```python
from build123d import *

# Parameters (mm, degrees)
SKETCH1_R             = 66.4845
BOSS_EXTRUDE1_DEPTH   = 11.43
CUT_EXTRUDE1_START    = -33.02
SKETCH3_W             = 41.275
SKETCH3_H             = 24.257
CUT_EXTRUDE1_DEPTH    = 46.278900076
SKETCH4_R             = 30.1625
CUT_EXTRUDE2_DEPTH    = 95.715481208
F_6_CLEARANCE_HOLE1_D = 3.7973
CIRPATTERN1_COUNT     = 5
CUT_EXTRUDE3_DEPTH    = 95.715481208
SKETCH9_W             = 90.169443187
SKETCH9_H             = 19.134747519
CUT_EXTRUDE4_DEPTH    = 82.281975988
CUT_EXTRUDE5_DEPTH    = 73.517528625


with BuildPart() as part:
    # Sketch1 → Boss-Extrude1 (new body)
    with BuildSketch(Plane.XY):
        Circle(SKETCH1_R)
    extrude(amount=BOSS_EXTRUDE1_DEPTH)

    # Sketch3 → Cut-Extrude1 (cut)
    with BuildSketch(Plane(origin=(0, 10.998843101, -24.703806075), x_dir=(1, 0, 0), z_dir=(0, -0.40673664307580104, 0.9135454576426005)).offset(CUT_EXTRUDE1_START)):
        with Locations((6.90118, 37.673412979)):
            Rectangle(SKETCH3_W, SKETCH3_H)
    cut_extrude1 = extrude(amount=CUT_EXTRUDE1_DEPTH, mode=Mode.SUBTRACT)

    # Sketch4 → Cut-Extrude2 (cut, through all)
    with BuildSketch(Plane(origin=(0, 0, 0), x_dir=(-1, 0, 0), z_dir=(0, 0, -1))):
        Circle(SKETCH4_R)
    extrude(amount=-CUT_EXTRUDE2_DEPTH, mode=Mode.SUBTRACT)

    # #6 Clearance Hole1 (through all)
    with Locations(Plane(origin=(0, 0, 0), x_dir=(-1, 0, 0), z_dir=(0, 0, -1))):
        with Locations((-32.61868, 45.624980685), (18.81632, 45.624980685)):
            f_6_clearance_hole1 = Hole(F_6_CLEARANCE_HOLE1_D / 2)

    # CirPattern1: Cut-Extrude1, #6 Clearance Hole1 ×5 about axis
    cirpattern1_axis = Axis((0, 0, 0), (0, 0, 1))
    add([cut_extrude1.rotate(cirpattern1_axis, i * 360 / CIRPATTERN1_COUNT) for i in range(1, CIRPATTERN1_COUNT)], mode=Mode.SUBTRACT)
    add([f_6_clearance_hole1.rotate(cirpattern1_axis, i * 360 / CIRPATTERN1_COUNT) for i in range(1, CIRPATTERN1_COUNT)], mode=Mode.SUBTRACT)

    # Sketch5 → Cut-Extrude3 (cut, through all)
    with BuildSketch(Plane(origin=(0, 0, 0), x_dir=(-1, 0, 0), z_dir=(0, 0, -1))):
        with BuildLine():
            Line((-45.34231997, 48.623685175), (0, 0))
            Line((0, 0), (32.232325197, 58.148653919))
            ThreePointArc((32.232325197, 58.148653919), (8.102422362, -65.988934619), (-45.34231997, 48.623685175))
        make_face()
    extrude(amount=-CUT_EXTRUDE3_DEPTH, mode=Mode.SUBTRACT)

    # Sketch9 → Cut-Extrude4 (cut, through all)
    with BuildSketch(Plane.XY.offset(11.43)):
        Polygon((-20.16444413, 36.377620169), (33.922679606, 36.377620169), (0, 0), align=None)
        with Locations((9.105457651, 64.994993929)):
            Rectangle(SKETCH9_W, SKETCH9_H)
    extrude(amount=-CUT_EXTRUDE4_DEPTH, mode=Mode.SUBTRACT)

    # Sketch10 → Cut-Extrude5 (cut, through all)
    with BuildSketch(Plane.XY.offset(11.43)):
        with BuildLine():
            Line((-20.16444413, 36.377620169), (-37.32827131, 36.377620169))
            Line((-37.32827131, 36.377620169), (-35.716510793, 61.307238028))
            Line((-35.716510793, 61.307238028), (-20.16444413, 55.427620169))
            ThreePointArc((-20.16444413, 55.427620169), (-22.716660188, 45.902620169), (-20.16444413, 36.377620169))
        make_face()
        with BuildLine():
            Line((33.922679606, 36.377620169), (47.375187835, 33.198791646))
            Line((47.375187835, 33.198791646), (54.157749271, 61.901964171))
            Line((54.157749271, 61.901964171), (32.96596662, 55.427620169))
            ThreePointArc((32.96596662, 55.427620169), (36.00025444, 46.03098199), (33.922679606, 36.377620169))
        make_face()
    extrude(amount=-CUT_EXTRUDE5_DEPTH, mode=Mode.SUBTRACT)


solid = part.part
```
The listing builds one solid part. Answer for the finished solid, in the listing's coordinates (mm). A direction names the side the tool comes from. Give positions to 0.01 mm unless a question says otherwise; leave off trailing zeros. Order: outer loops, then holes, each group sorted by start corner. A loop starts at its lowest first (then second) coordinate and runs counter-clockwise, first axis right, second up. Notation, with made-up numbers: (-13, -12.5) - (11, -12.5) arc R20 ccw to (11, 25.5) - close; hole circle Ø1 at (44, 88). An arc over 180 degrees is marked (long way). Answer in a Markdown table with one row per item. Add a question column.
Q1. The part is cut by section D-D (z = 8.25). Determine the outline of the cut face in (x, y).
Q2. For a pull along Z with two mould halves and no side action, classify faces 1 (the flat face through (9, 55, 0)), 2 (the flat face through (6, 46, 11.43)), 3 (the cylindrical face through (33.639, 47.226, 5.795)) as released by +Z, released by -Z, zero draft, split by the parting line, or undercut.
Q3. The part is cut by section C-C (z = 3). Determine the outline of the cut face in (x, y), then the cut area to 3 significant figures.
Q4. The part is cut by section A-A (y = 45). Determine the outline of the cut face in (x, z), then the cut area to 3 significant figures.
Q5. The part is cut by section B-B (x = -3.5). Determine the outline of the cut face in (y, z).
Q6. Find the intervals of material crossed by line 1 along X through (y, z) = (44.25, 9.25); line 2 along X through (y, z) = (45.25, 0.5); line 3 along Y through (x, z) = (-9, 2.25), in increasing order. Write a range as [from, to].
Q7. Given P1, Ø1, axis at x = -11, y = 40, coming from the -Z side; P2, Ø6, axis at y = 41, z = 2.5, coming from the -X side, each flat-ended and moving along its own axis, determine where each tip first touches the part or whether it passes through.
Q8. Which of the six approach directions +Z, -Z, +X, -X, +Y, -Y give full straight-line access (tool end or side, diameter ignored) to faces 4 (the cylindrical face through (-22.71, 46.37, 5.8)), 5 (the flat face through (6.61, 43.84, 4.43))?
Determined:
| question | item | result |
|---|---|---|
| 1 | outline | (-20.49, 36.96) - (-20.16, 36.38) - (33.92, 36.38) arc R19.05 ccw to (32.97, 55.43) - (-20.16, 55.43) arc R19.05 ccw to start; hole circle Ø3.8 at (-18.82, 45.62); hole circle Ø3.8 at (32.62, 45.62) |
| 2 | face 1 | released by -Z |
| 2 | face 2 | released by +Z |
| 2 | face 3 | zero draft |
| 3 | outline | (-20.49, 36.96) - (-20.16, 36.38) - (33.92, 36.38) arc R19.05 ccw to (32.97, 55.43) - (-20.16, 55.43) arc R19.05 ccw to start; hole circle Ø3.8 at (-18.82, 45.62); hole (-13.74, 40.62) - (27.54, 40.62) - (27.54, 53.18) - (-13.74, 53.18) - close; hole circle Ø3.8 at (32.62, 45.62) |
| 3 | area | 546 mm² |
| 4 | outline | (-22.7, 0) - (-20.61, 0) - (-20.61, 11.43) - (-22.7, 11.43) - close; (-17.02, 0) - (-13.74, 0) - (-13.74, 4.95) - (27.54, 4.95) - (27.54, 0) - (30.83, 0) - (30.83, 11.43) - (-17.02, 11.43) - close; (34.41, 0) - (36.02, 0) - (36.02, 11.43) - (34.41, 11.43) - close |
| 4 | area | 385 mm² |
| 5 | outline | (36.38, 1.11) - (51.1, 7.67) - (54.51, 0) - (55.43, 0) - (55.43, 11.43) - (36.38, 11.43) - close |
| 6 | line 1 | x = [-22.64, -20.13], [-17.51, 31.31], [33.93, 36.01] |
| 6 | line 2 | x = [-22.71, -20.68], [-16.96, -13.74], [27.54, 30.76], [34.48, 36.02] |
| 6 | line 3 | y = [36.38, 38.94], [53.51, 55.43] |
| 7 | P1 | stops at z = 2.5 |
| 7 | P2 | stops at x = -22.62 |
| 8 | face 4 | +Z, -Z, -X |
| 8 | face 5 | -Z |
